Geometry: final body of the model. Coordinates: model frame, mm. A direction names the side the tool comes from. Give positions to 0.01 mm unless a question says otherwise; leave off trailing zeros. Write each loop counter-clockwise with the first axis right and the second up, starting at its lowest first coordinate (ties: lowest second). Pieces come first, ordered by that corner, then holes. Notation, with made-up numbers: (18, -25.5) -> (59, -25.5) arc R30 ccw to (59, -2.5) -> close; hole circle Ø5 at (28.5, 35.25). An arc over 180 degrees is marked (long way). Use CSV: the item, a comma, the result in double quotes. Start each with the question number.
1) Contact query for flat-ended pins moving along their axis: P1, Ø0.5, axis at x = 56, y = -0.5, coming from the +Z side; P2, Ø2.5, axis at y = -5.5, z = -1.5, coming from the +X side; P3, Ø23.5, axis at x = 41.5, z = 11.5, coming from the -Y side. Output: stop coordinate, or through.
2) Set-up query: faces 1 (the face through (65, -6, -5.28)), 2 (the face through (68, -6, 0)), 3 (the face through (-3, 0, -1)), 4 (the face through (65, -6, 5.28)), 5 (the face through (63, -6, 0)). Return all of +Z, -Z, +X, -X, +Y, -Y with unobstructed straight access to the full face (end or side cutting, diameter ignored); none if empty.
3) Section B-B (x = -7). Output: boundary loops of the cut face in (y, z).
4) Material intervals for line 1 (Y direction, x = -19, z = -25); line 2 (Z direction, x = 65, y = -5.75); line 3 (Z direction, x = 34.5, y = -0.75), sorted ascending. Write a range as [from, to].
5) Section A-A (z = 3). Output: boundary loops of the cut face in (x, y).
6) Section C-C (y = -3.25). Output: boundary loops of the cut face in (x, z).
```python
from build123d import *

# Parameters (mm, degrees)
SKETCH1_W           = 60
SKETCH1_H           = 78
SKETCH1_W_2         = 40
SKETCH1_H_2         = 15
BOSS_EXTRUDE1_DEPTH = 1.6
SKETCH2_W           = 5
SKETCH2_H           = 10.56
BOSS_EXTRUDE2_DEPTH = 8


with BuildPart() as part:
    # Sketch1 → Boss-Extrude1 (new body)
    with BuildSketch(Plane(origin=(0, 0, 0), x_dir=(1, 0, 0), z_dir=(0, 1, 0))):
        Rectangle(SKETCH1_W, SKETCH1_H)
        with Locations((50, 0)):
            Rectangle(SKETCH1_W_2, SKETCH1_H_2)
    extrude(amount=-BOSS_EXTRUDE1_DEPTH)

    # Sketch2 → Boss-Extrude2 (add)
    with BuildSketch(Plane.XZ.offset(1.6)):
        with Locations((65.5, 0)):
            Rectangle(SKETCH2_W, SKETCH2_H)
    extrude(amount=BOSS_EXTRUDE2_DEPTH)


solid = part.part
```
Answers follow:
1,P1,"stops at z = 7.5"
1,P2,"stops at x = 68"
1,P3,"stops at y = -1.6"
2,face 1,"-Z, +X, -X, -Y"
2,face 2,"+Z, -Z, +X, -Y"
2,face 3,"+Z, -Z, +X, -X, +Y"
2,face 4,"+Z, +X, -X, -Y"
2,face 5,"+Z, -Z, -X, -Y"
3,outline,"(-1.6, -39) -> (0, -39) -> (0, 39) -> (-1.6, 39) -> close"
4,line 1,"y = [-1.6, 0]"
4,line 2,"z = [-5.28, 5.28]"
4,line 3,"z = [-7.5, 7.5]"
5,outline,"(-30, -1.6) -> (63, -1.6) -> (63, -9.6) -> (68, -9.6) -> (68, -1.6) -> (70, -1.6) -> (70, 0) -> (-30, 0) -> close"
6,outline,"(63, -5.28) -> (68, -5.28) -> (68, 5.28) -> (63, 5.28) -> close"
